Here's the drawing with two shaded views (mm, measured from the low corner). I have some questions. A direction names the side the tool comes from. Give positions to 0.01 mm unless a question says otherwise; leave off trailing zeros. Write each loop counter-clockwise with the first axis right and the second up, starting at its lowest first coordinate (ties: lowest second). Pieces come first, ordered by that corner, then holes. Notation, with made-up numbers: M 70,76.25 L 98,76.25 A24 cw 98,102.25 Z; hole C -29,-32.75 d7. An arc over 180 degrees is marked long. Answer as a JSON object with one key per item and string values. Group by question number.
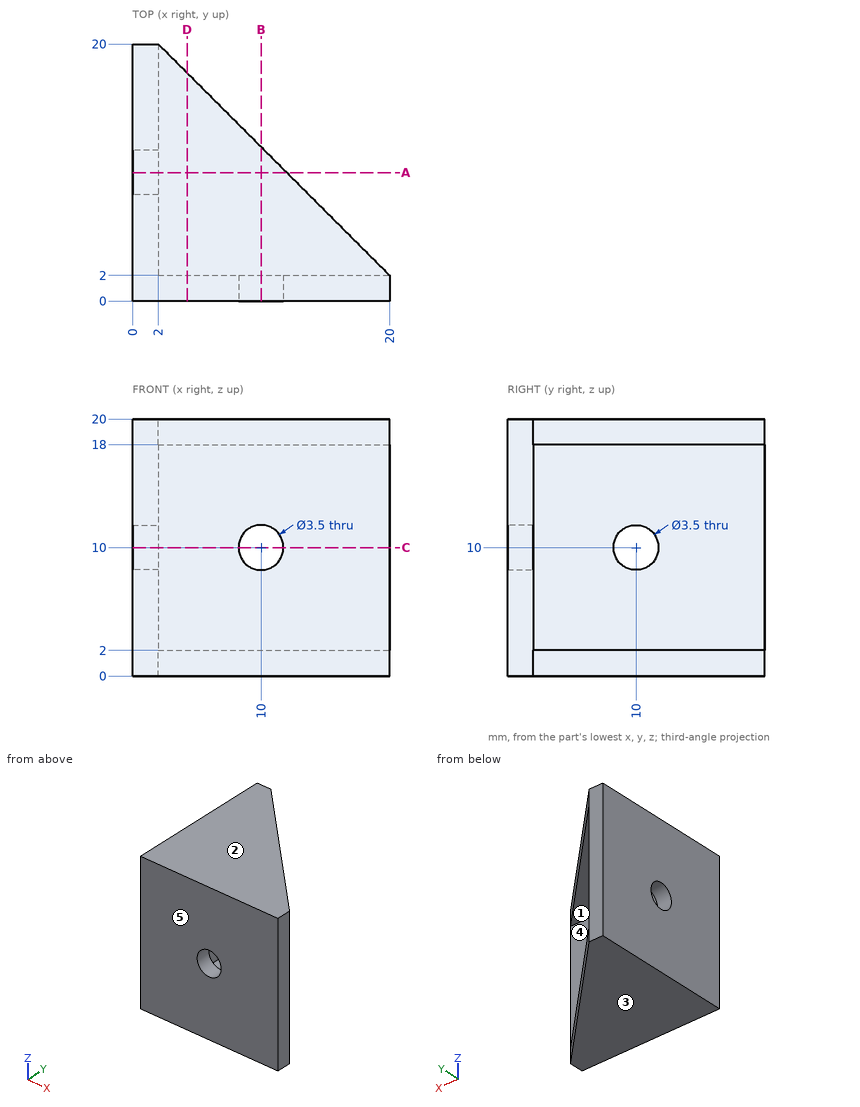
1) I'm going to push flat-ended pins straight in: pin 1 (5 mm diameter, centred on y = 10.5, z = 9, fed in from +X); pin 2 (10 mm diameter, centred on x = 10, z = 11, fed in from +Y). Where does each tip first touch, or does it pass through?
2) Please list where these lines run through material, in increasing order: line 1 along Z through (x, y) = (18, 2.25); line 2 along X through (y, z) = (1.2, 10). Write a range as from..to.
3) If we section it at A-A, the plane y = 10: List the corners of the cut face in (x, z) for me.
4) We'd pull the mould along Z, two halves only. Please class the marked faces 1, 2 and 3: released by +Z, released by -Z, zero draft, split by the parting line, or undercut.
5) For the marked faces 4 and 5, which set-ups out of +Z, -Z, +X, -X, +Y, -Y let a thin tool reach every point of the face, with its end or its side?
6) If we section it at C-C, the plane z = 10: List the corners of the cut face in (x, y) for me.
7) If we section it at D-D, the plane x = 4.25: List the corners of the cut face in (y, z) for me, plus the area to 3 significant figures.
Taken from the geometry:
{
 "1": {"pin 1": "x = 2", "pin 2": "y = 2"},
 "2": {"line 1": "0..2, 18..20", "line 2": "0..8.25, 11.75..20"},
 "3": {"outline": "M 0,0 L 12,0 L 12,2 L 2,2 L 2,8.25 L 0,8.25 Z; M 0,11.75 L 2,11.75 L 2,18 L 12,18 L 12,20 L 0,20 Z"},
 "4": {"face 1": "undercut", "face 2": "released by +Z", "face 3": "released by -Z"},
 "5": {"face 4": "+X, +Y", "face 5": "+Z, -Z, +X, -X, -Y"},
 "6": {"outline": "M 0,0 L 8.25,0 L 8.25,2 L 2,2 L 2,8.25 L 0,8.25 Z; M 0,11.75 L 2,11.75 L 2,20 L 0,20 Z; M 11.75,0 L 20,0 L 20,2 L 11.75,2 Z"},
 "7": {"outline": "M 0,0 L 17.75,0 L 17.75,2 L 2,2 L 2,18 L 17.75,18 L 17.75,20 L 0,20 Z", "area": "103 mm²"}
}
